The listing builds one solid part. Answer for the finished solid, in the listing's coordinates (mm). A direction names the side the tool comes from. Round coordinates to 2 decimals unless told otherwise and drop trailing zeros. Order: outer loops, then holes, each group sorted by start corner. A loop starts at its lowest first (then second) coordinate and runs counter-clockwise, first axis right, second up. Notation, with made-up numbers: M 47,-36 L 76,-36 A24 ccw 76,-9 Z; hole C -15,10 d7. An arc over 180 degrees is marked long. Put each result on its own line as item: value. Start each with the question number.
1. This flat-tipped pin is pushed along its axis until it touches: pin 1 Ø1.8 at (x, y) = (3.4, 3.5) entering from -Z. Where does it stop, or does it pass through?
2. The part is cut by section A-A (z = 3.5). Give the vertices of the cut face in (x, y).
3. Consider line 1 (Y direction, x = 3.5, z = 3.5); line 2 (Z direction, x = 2.5, y = 3.25); line 3 (X direction, y = 0.75, z = -1.5). Determine where each line is inside the solid, lowest interval first.
4. The part is cut by section C-C (y = 0.68). Give the vertices of the cut face in (x, z), then the cut area to 3 significant figures.
5. The mould has two halves that part along Y. Classify faces 3 (the face through (3, 0, 2)), 4 (the face through (3, 7, 2)), 5 (the face through (3.25, 4, 4)), 6 (the face through (3, 4, 0)): +Y half, -Y half, draft (parallel to the pull), parting line (faces both ways), or undercut.
6. The part is cut by section D-D (z = -1.5). Give the vertices of the cut face in (x, y).
7. Which of the six approach directions +Z, -Z, +X, -X, +Y, -Y give full straight-line access (tool end or side, diameter ignored) to faces 1 (the face through (0, 4, 2)), 2 (the face through (3.25, 3, 4))?
Autodesk Inventor part; units mm, degrees
ref_plane "YZ Plane" through (0, 0, 0) normal (1, 0, 0) x (0, 1, 0)
ref_plane "XZ Plane" through (0, 0, 0) normal (0, 1, 0) x (-1, 0, 0)
ref_plane "XY Plane" through (0, 0, 0) normal (0, 0, 1) x (1, 0, 0)
sketch "Skizze1" plane through (0, 0, 0) normal (0, 0, 1) x (1, 0, 0)
  line L0 (0, 0) -> (6.8, 0)
  line L1 (6.8, 0) -> (6.8, 7)
  line L2 (6.8, 7) -> (0, 7)
  line L3 (0, 7) -> (0, 0)
  dimension "d0" = 6.8
  dimension "d1" = 7
extrude "Extrusion1" add sketch "Skizze1" along normal blind 4.8
sketch "Skizze2" plane through (0, 0, 4.8) normal (0, 0, 1) x (1, 0, 0)
  line L0 (0, 0) -> (6.8, 0) construction
  line L1 (6.8, 0) -> (6.8, 7) construction
  line L2 (6.8, 7) -> (0, 7) construction
  line L3 (0, 7) -> (0, 0) construction
  circle A0 centre (3.4, 3.5) radius 1.5
  point P0 (0, 3.5)
  point P1 (3.4, 7)
  dimension "d4" = 3
extrude "Extrusion2" cut sketch "Skizze2" against normal blind 0.01
sketch "Skizze3" plane through (3.4, 3.5, 4.79) normal (0, 0, 1) x (1, 0, 0)
  line L0 (-0.15, 1.4925) -> (0.15, 1.4925)
  line L1 (0.15, -1.4925) -> (-0.15, -1.4925)
  line L2 (1.4925, 0.15) -> (1.4925, -0.15)
  line L3 (-1.4925, -0.15) -> (-1.4925, 0.15)
  line L4 (-1.4925, 0.15) -> (-0.15, 0.15)
  line L5 (0.15, 0.15) -> (1.4925, 0.15)
  line L6 (0.15, 1.4925) -> (0.15, 0.15)
  line L7 (0.15, -0.15) -> (0.15, -1.4925)
  line L8 (-0.15, -1.4925) -> (-0.15, -0.15)
  line L9 (-0.15, 0.15) -> (-0.15, 1.4925)
  line L10 (1.4925, -0.15) -> (0.15, -0.15)
  line L11 (-0.15, -0.15) -> (-1.4925, -0.15)
  line L12 (0, 1.4925) -> (0, -1.4925) construction
  line L13 (-1.4925, 0) -> (1.4925, 0) construction
  circle A0 centre (0, 0) radius 1.5 construction
  point P0 (-3.4, -3.5)
  dimension "d7" = 0.3
extrude "Extrusion3" cut sketch "Skizze3" against normal blind 1.5
sketch "Skizze4" plane through (0, 0, 0) normal (0, 0, -1) x (-1, 0, 0)
  circle A0 centre (-0.86, 3.22) radius 0.25
  circle A1 centre (-5.94, 3.22) radius 0.25
  circle A2 centre (-3.4, 0.68) radius 0.25
  line L0 (0, 0) -> (-6.8, 0) construction
  line L1 (-3.4, 0) -> (-3.4, 7) construction
  line L2 (-6.8, 7) -> (0, 7) construction
  dimension "d10" = 0.5
  dimension "d11" = 5.08
  dimension "d12" = 2.54
  dimension "d13" = 0.68
extrude "Extrusion4" add sketch "Skizze4" along normal blind 2.5
properties part number "Poti" material "PBT-Kunststoff"
Resolved:
1. pin 1: z = 0
2. outline: M 0,0 L 6.8,0 L 6.8,7 L 0,7 Z; hole M 1.91,3.35 L 3.25,3.35 L 3.25,2.01 L 3.55,2.01 L 3.55,3.35 L 4.89,3.35 L 4.89,3.65 L 3.55,3.65 L 3.55,4.99 L 3.25,4.99 L 3.25,3.65 L 1.91,3.65 Z
3. line 1: 0 to 2.01, 4.99 to 7
3. line 2: 0 to 4.79
3. line 3: 3.16 to 3.64
4. outline: M 0,0 L 3.15,0 L 3.15,-2.5 L 3.65,-2.5 L 3.65,0 L 6.8,0 L 6.8,4.8 L 0,4.8 Z
4. area: 33.9 mm2
5. face 3: -Y half
5. face 4: +Y half
5. face 5: undercut
5. face 6: draft
6. outline: C 0.86,3.22 d0.5; C 3.4,0.68 d0.5; C 5.94,3.22 d0.5
7. face 1: +Z, -Z, -X, +Y, -Y
7. face 2: +Z
